Can you work these out from the model? Positions are in its coordinate system, mm. Face numbers are marked on the shaded views. A direction names the side the tool comes from. Coordinates: 2 decimals unless noted, no trailing zeros. Loops run counter-clockwise (first coordinate to the right, second up) from the corner with the lowest first, then second, coordinate; pieces in that order, holes last.
```python
from build123d import *

# Parameters (mm, degrees)
BOSS_EXTRUDE1_DEPTH = 1.5
CUT_EXTRUDE1_DEPTH  = 2
SKETCH3_R           = 4
CUT_EXTRUDE2_DEPTH  = 2
SKETCH4_R           = 20
CUT_EXTRUDE3_DEPTH  = 0.5
FILLET1_R           = 1
SKETCH5_R           = 22
BOSS_EXTRUDE2_DEPTH = 3
SKETCH7_R           = 7.5
BOSS_EXTRUDE4_DEPTH = 1.5
SKETCH8_R           = 22
BOSS_EXTRUDE5_DEPTH = 7
SKETCH9_R           = 8
SKETCH9_R_2         = 6.5
CUT_EXTRUDE4_DEPTH  = 3
FILLET4_R           = 3
SKETCH10_R          = 46.144445172
SKETCH10_R_2        = 20.866025404
CUT_EXTRUDE5_DEPTH  = 6
CUT_EXTRUDE6_START  = -10
SKETCH12_R          = 20.866025404
SKETCH12_R_2        = 6.5
CUT_EXTRUDE6_DEPTH  = 10
FILLET5_R           = 4
SKETCH13_R          = 8.896552767
SKETCH13_R_2        = 4.5
CUT_EXTRUDE7_DEPTH  = 4
SKETCH14_R          = 4
BOSS_EXTRUDE7_DEPTH = 18


# Some blends are built 0.0001 mm under size
with BuildPart() as part:
    # Sketch1 → Boss-Extrude1 (new body)
    with BuildSketch(Plane(origin=(0, 0, 0), x_dir=(1, 0, 0), z_dir=(0, 1, 0))):
        with BuildLine():
            Line((-20.5, -35), (20.5, -35))
            ThreePointArc((20.5, -35), (24.035533906, -33.535533906), (25.5, -30))
            Line((25.5, -30), (25.5, 30))
            ThreePointArc((25.5, 30), (24.035533906, 33.535533906), (20.5, 35))
            Line((20.5, 35), (-20.5, 35))
            ThreePointArc((-20.5, 35), (-24.035533906, 33.535533906), (-25.5, 30))
            Line((-25.5, 30), (-25.5, -30))
            ThreePointArc((-25.5, -30), (-24.035533906, -33.535533906), (-20.5, -35))
        make_face()
    extrude(amount=BOSS_EXTRUDE1_DEPTH)

    # Sketch2 → Cut-Extrude1 (cut)
    with BuildSketch(Plane(origin=(0, 1.5, 0), x_dir=(1, 0, 0), z_dir=(0, 1, 0))):
        with BuildLine():
            Line((-21.5, 24.5), (-21.5, 28.5))
            ThreePointArc((-21.5, 28.5), (-17.5, 32.5), (-13.5, 28.5))
            Line((-13.5, 28.5), (-13.5, 24.5))
            ThreePointArc((-13.5, 24.5), (-17.5, 20.5), (-21.5, 24.5))
        make_face()
        with BuildLine():
            Line((13.5, 24.5), (13.5, 28.5))
            ThreePointArc((13.5, 28.5), (17.5, 32.5), (21.5, 28.5))
            Line((21.5, 28.5), (21.5, 24.5))
            ThreePointArc((21.5, 24.5), (17.5, 20.5), (13.5, 24.5))
        make_face()
    cut_extrude1 = extrude(amount=-CUT_EXTRUDE1_DEPTH, mode=Mode.SUBTRACT)

    # Mirror1: Cut-Extrude1 across plane
    add(cut_extrude1.mirror(Plane.XY), mode=Mode.SUBTRACT)

    # Sketch3 → Cut-Extrude2 (cut)
    with BuildSketch(Plane(origin=(0, 1.5, 0), x_dir=(1, 0, 0), z_dir=(0, 1, 0))):
        with Locations(Location((0, 0, 0), (0, 0, 270))):
            Circle(SKETCH3_R)
    extrude(amount=-CUT_EXTRUDE2_DEPTH, mode=Mode.SUBTRACT)

    # Sketch4 → Cut-Extrude3 (cut)
    with BuildSketch(Plane(origin=(0, 1.5, 0), x_dir=(1, 0, 0), z_dir=(0, 1, 0))):
        with Locations(Location((0, 0, 0), (0, 0, 270))):
            Circle(SKETCH4_R)
    extrude(amount=-CUT_EXTRUDE3_DEPTH, mode=Mode.SUBTRACT)

    # Fillet1
    # the kernel refuses this fillet: 1 mm, written as the material it takes off along each edge
    with BuildSketch(Plane(origin=(0, 1.5, 0), x_dir=(0, 0, 1), z_dir=(-1, 0, 0))) as fillet1_piece_1:
        with BuildLine():
            CenterArc((20.866025404, -1), FILLET1_R, 90, 60)
            Line((20, -0.5), (19.982679492, -0.49))
            ThreePointArc((19.982679492, -0.49), (19.98, -0.25), (19.98, 0))
            Line((19.98, 0), (20, 0.02))
            Line((20, 0.02), (20.866025404, 0.02))
            Line((20.866025404, 0.02), (20.866025404, 0))
        make_face()
    revolve(axis=Axis((0, 1.5, 0), (0, 1, 0)), mode=Mode.SUBTRACT)

    # Sketch5 → Boss-Extrude2 (add)
    with BuildSketch(Plane.XZ):
        with Locations(Location((0, 0, 0), (0, 0, 270))):
            Circle(SKETCH5_R)
    extrude(amount=BOSS_EXTRUDE2_DEPTH)

    # Sketch7 → Boss-Extrude4 (add)
    with BuildSketch(Plane.XZ.offset(3)):
        with Locations(Location((0, 0, 0), (0, 0, 270))):
            Circle(SKETCH7_R)
    extrude(amount=BOSS_EXTRUDE4_DEPTH)

    # Sketch8 → Boss-Extrude5 (add)
    with BuildSketch(Plane.XZ.offset(4.5)):
        with Locations(Location((0, 0, 0), (0, 0, 270))):
            Circle(SKETCH8_R)
    extrude(amount=BOSS_EXTRUDE5_DEPTH)

    # Sketch9 → Cut-Extrude4 (cut)
    with BuildSketch(Plane(origin=(0, 1, 0), x_dir=(1, 0, 0), z_dir=(0, 1, 0))):
        with Locations(Location((0, 0, 0), (0, 0, 270))):
            Circle(SKETCH9_R)
        with Locations(Location((0, 0, 0), (0, 0, 270))):
            Circle(SKETCH9_R_2, mode=Mode.SUBTRACT)
    extrude(amount=-CUT_EXTRUDE4_DEPTH, mode=Mode.SUBTRACT)

    # Fillet4
    fillet4_edges = [part.edges().sort_by_distance(p)[0] for p in [
        (0, 1, -8),
    ]]
    fillet(fillet4_edges, radius=FILLET4_R - 0.0001)  # a hair under: the kernel refuses the full size

    # Sketch10 → Cut-Extrude5 (cut)
    with BuildSketch(Plane(origin=(0, 1.5, 0), x_dir=(1, 0, 0), z_dir=(0, 1, 0))):
        Circle(SKETCH10_R)
        with Locations(Location((0, 0, 0), (0, 0, 270))):
            Circle(SKETCH10_R_2, mode=Mode.SUBTRACT)
    extrude(amount=-CUT_EXTRUDE5_DEPTH, mode=Mode.SUBTRACT)

    # Sketch12 → Cut-Extrude6 (cut)
    with BuildSketch(Plane.XZ.offset(3).offset(CUT_EXTRUDE6_START)):
        Circle(SKETCH12_R)
        with Locations(Location((0, 0, 0), (0, 0, 90))):
            Circle(SKETCH12_R_2, mode=Mode.SUBTRACT)
    extrude(amount=CUT_EXTRUDE6_DEPTH, mode=Mode.SUBTRACT)

    # Fillet5
    fillet5_edges = [part.edges().sort_by_distance(p)[0] for p in [
        (0, -4.5, 22),
    ]]
    fillet(fillet5_edges, radius=FILLET5_R)

    # Sketch13 → Cut-Extrude7 (cut)
    with BuildSketch(Plane(origin=(0, 1, 0), x_dir=(1, 0, 0), z_dir=(0, 1, 0))):
        Circle(SKETCH13_R)
        with Locations(Location((0, 0, 0), (0, 0, 270))):
            Circle(SKETCH13_R_2, mode=Mode.SUBTRACT)
    extrude(amount=-CUT_EXTRUDE7_DEPTH, mode=Mode.SUBTRACT)

    # Sketch14 → Boss-Extrude7 (add)
    with BuildSketch(Plane(origin=(0, 0, 0), x_dir=(1, 0, 0), z_dir=(0, 1, 0))):
        with Locations(Location((0, 0, 0), (0, 0, 270))):
            Circle(SKETCH14_R)
    extrude(amount=-BOSS_EXTRUDE7_DEPTH)


solid = part.part
```
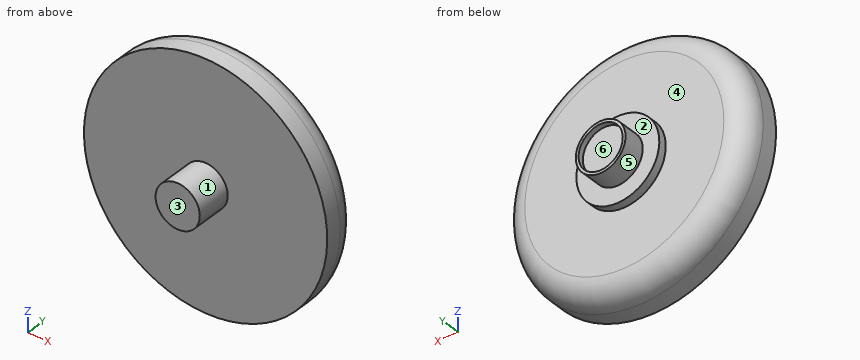
Item 1: Suppose I cut it at B-B, the plane z = 0. Please give me the cut outline in (x, y).
Results are:
outline: (-22, -11.5) - (-4, -11.5) - (-4, -18) - (4, -18) - (4, -11.5) - (22, -11.5) - (22, -8.5) arc R4 ccw to (18, -4.5) - (7.5, -4.5) - (7.5, -3) - (4.5, -3) - (4.5, 1) - (4, 1) - (4, 0) - (-4, 0) - (-4, 1) - (-4.5, 1) - (-4.5, -3) - (-7.5, -3) - (-7.5, -4.5) - (-18, -4.5) arc R4 ccw to (-22, -8.5) - close
Item 2: I'm going to push flat-ended pins straight in: P1, Ø3, axis at x = 15.5, z = -6, coming from the -Y side; P2, Ø12, axis at x = -1.5, z = 3, coming from the +Y side; P3, Ø10, axis at x = 6, y = -12.5, coming from the +Z side; P4, Ø4, axis at x = 17, y = -1, coming from the -Z side. Where does each tip first touch, or does it pass through?
Results are:
P1: stops at y = -11.5
P2: stops at y = 1
P3: stops at z = 21.97
P4: passes through
Item 3: On a 3-axis mill with a long thin cutter (end or side, diameter ignored), from which of +Z, -Z, +X, -X, +Y, -Y can I reach the whole of each face in a straight line? I mean the marked faces 1, 2 and 3. Say none if no direction works.
Results are:
face 1: -Y
face 2: +Y
face 3: +Z, -Z, +X, -X, -Y
Item 4: Suppose I cut it at D-D, the plane y = -7. Please give me the cut outline in (x, z), plus the area to 3 significant figures.
Results are:
outline: circle Ø43.42 at (0, 0)
area: 1,480 mm2
Item 5: Suppose I cut it at C-C, the plane y = -15.5. Please give me the cut outline in (x, z).
Results are:
outline: circle Ø8 at (0, 0)
Item 6: Suppose I cut it at A-A, the plane x = 0. Please give me the cut outline in (y, z).
Results are:
outline: (-18, -4) - (-11.5, -4) - (-11.5, -22) - (-8.5, -22) arc R4 ccw to (-4.5, -18) - (-4.5, -7.5) - (-3, -7.5) - (-3, -4.5) - (1, -4.5) - (1, -4) - (0, -4) - (0, 4) - (1, 4) - (1, 4.5) - (-3, 4.5) - (-3, 7.5) - (-4.5, 7.5) - (-4.5, 18) arc R4 ccw to (-8.5, 22) - (-11.5, 22) - (-11.5, 4) - (-18, 4) - close
Item 7: We'd pull the mould along X, two halves only. Please class the marked faces 4, 5 and 6: +X half, -X half, draft (parallel to the pull), parting line (faces both ways), or undercut.
Results are:
face 4: draft
face 5: parting line
face 6: undercut
Item 8: I need wall thicknesses on line 1 along X through (y, z) = (0.6, 0); line 2 along Y through (x, z) = (3, 9); line 3 along X through (y, z) = (-11, 0). Which ranges of each line are inside material? Lowest first, please.
Results are:
line 1: x = -4.5 to -4, 4 to 4.5
line 2: y = -11.5 to -4.5
line 3: x = -22 to 22
